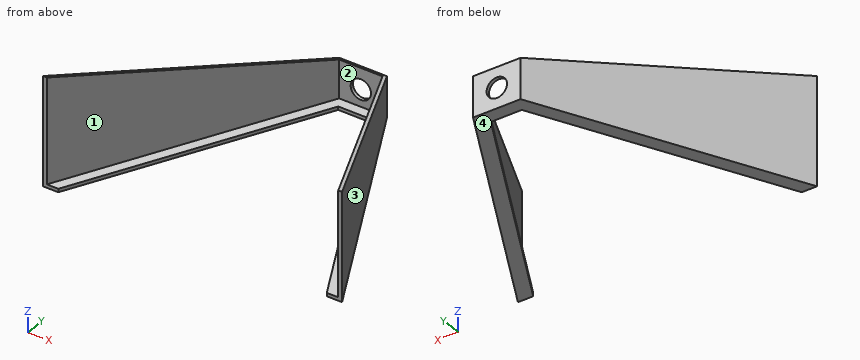
from build123d import *

# Parameters (mm, degrees)
BOSS_EXTRUDE1_DEPTH     = 203.2
CUT_EXTRUDE1_DEPTH      = 280.4
CUT_EXTRUDE1_DEPTH_BACK = 280.4
SHELL1_T                = -6.35
CUT_EXTRUDE2_DEPTH      = 204.2
SKETCH4_R               = 19.05
CUT_EXTRUDE3_DEPTH      = 458.2


with BuildPart() as part:
    # Sketch1 → Boss-Extrude1 (new body)
    with BuildSketch(Plane.XY):
        Polygon((-279.4, 0), (-44.45, 457.2), (44.45, 457.2), (279.4, 0), align=None)
    extrude(amount=BOSS_EXTRUDE1_DEPTH)

    # Sketch2 → Cut-Extrude1 (cut, two sides)
    with BuildSketch(Plane(origin=(0, 0, 0), x_dir=(0, 0, -1), z_dir=(1, 0, 0))) as cut_extrude1_sk:
        Polygon((-203.2, 0), (-76.2, 457.2), (-203.2, 457.2), align=None)
    extrude(amount=CUT_EXTRUDE1_DEPTH, mode=Mode.SUBTRACT)
    extrude(cut_extrude1_sk.sketch, amount=-CUT_EXTRUDE1_DEPTH_BACK, mode=Mode.SUBTRACT)

    # Shell1
    shell1_openings = [part.faces().sort_by_distance(p)[0] for p in [
        (0, 228.6, 139.7),
        (0, 0, 101.6),
    ]]
    offset(amount=SHELL1_T, openings=shell1_openings, kind=Kind.INTERSECTION)

    # Sketch3 → Cut-Extrude2 (cut, through all)
    with BuildSketch(Plane(origin=(0, 0, 0), x_dir=(-1, 0, 0), z_dir=(0, 0, -1))):
        Polygon((250.842426439, 0), (28.945204216, 431.8), (-28.945204216, 431.8), (-250.842426439, 0), align=None)
    extrude(amount=-CUT_EXTRUDE2_DEPTH, mode=Mode.SUBTRACT)

    # Sketch4 → Cut-Extrude3 (cut, through all)
    with BuildSketch(Plane(origin=(0, 457.2, 0), x_dir=(1, 0, 0), z_dir=(0, 1, 0))):
        with Locations((0, -38.1)):
            Circle(SKETCH4_R)
    extrude(amount=-CUT_EXTRUDE3_DEPTH, mode=Mode.SUBTRACT)


solid = part.part
CAD build for the part. Positions are in the model's coordinates, mm. Face numbers are marked on the shaded views. Give positions to 0.01 mm unless a question says otherwise; leave off trailing zeros. Write each loop counter-clockwise with the first axis right and the second up, starting at its lowest first coordinate (ties: lowest second). Pieces come first, ordered by that corner, then holes. Notation, with made-up numbers: (56, 73) -> (81, 73) arc R22 cw to (81, 80) -> close; hole circle Ø7 at (19.25, -3.5). An arc over 180 degrees is marked (long way). Return JSON: item names as keys, results as strings.
Item 1: Band-saw the part on B-B (y = 416). List the corners of the cut face in (x, z), then the cut area to 3 significant figures.
Answer below:
{"outline": "(-65.62, 0) -> (-37.06, 0) -> (-37.06, 6.35) -> (-58.48, 6.35) -> (-58.48, 87.64) -> (-65.62, 87.64) -> close; (37.06, 0) -> (65.62, 0) -> (65.62, 87.64) -> (58.48, 87.64) -> (58.48, 6.35) -> (37.06, 6.35) -> close", "area": "1,520 mm2"}
Item 2: Drill centre lines: probe 1 along X at (y, z) = (456.25, 38.1); probe 2 along Z at (x, y) = (0, 452.75); probe 3 along X at (y, z) = (129, 161). Where is each one in solid material? Low to high.
Answer below:
{"probe 1": "x = -44.94 to -19.05, 19.05 to 44.94", "probe 2": "z = 0 to 19.05, 57.15 to 77.44", "probe 3": "x = -213.11 to -205.97, 205.97 to 213.11"}
Item 3: Two-plate mould, pull along X, no slides. Class the marked faces 1, 2, 3 and 4: +X half, -X half, draft (parallel to the pull), parting line (faces both ways), or undercut.
Answer below:
{"face 1": "undercut", "face 2": "undercut", "face 3": "+X half", "face 4": "draft"}
Item 4: Band-saw the part on C-C (z = 38.1). List the corners of the cut face in (x, y), then the cut area to 3 significant figures.
Answer below:
{"outline": "(-279.4, 0) -> (-272.26, 0) -> (-40.57, 450.85) -> (-19.05, 450.85) -> (-19.05, 457.2) -> (-44.45, 457.2) -> close; (19.05, 450.85) -> (40.57, 450.85) -> (272.26, 0) -> (279.4, 0) -> (44.45, 457.2) -> (19.05, 457.2) -> close", "area": "6,780 mm2"}
Item 5: Band-saw the part on D-D (z = 65). List the corners of the cut face in (x, y), then the cut area to 3 significant figures.
Answer below:
{"outline": "(-279.4, 0) -> (-272.26, 0) -> (-40.57, 450.85) -> (40.57, 450.85) -> (272.26, 0) -> (279.4, 0) -> (44.45, 457.2) -> (-44.45, 457.2) -> close", "area": "7,020 mm2"}
Item 6: Drop flat-ended pins along their axis: pin 1 (10 mm diameter, centred on x = -165.5, z = 106.5, fed in from +Y); pin 2 (3 mm diameter, centred on x = -13.5, z = 2.5, fed in from -Y). Give the stop position or say it passes through.
Answer below:
{"pin 1": "stops at y = 231.37", "pin 2": "stops at y = 431.8"}
Item 7: Band-saw the part on A-A (x = 0). List the corners of the cut face in (y, z), then the cut area to 3 significant figures.
Answer below:
{"outline": "(431.8, 0) -> (457.2, 0) -> (457.2, 19.05) -> (450.85, 19.05) -> (450.85, 6.35) -> (431.8, 6.35) -> close; (450.85, 57.15) -> (457.2, 57.15) -> (457.2, 76.2) -> (450.85, 77.96) -> close", "area": "369 mm2"}
